Here's how the part is built. I have some questions about the finished solid (model axes, mm). Coordinates: 2 decimals unless noted, no trailing zeros. Order: outer loops, then holes, each group sorted by start corner. A loop starts at its lowest first (then second) coordinate and runs counter-clockwise, first axis right, second up. Notation, with made-up numbers: (16, -29) - (27, -29) arc R32 cw to (27, 0) - close; hole circle Ø11 at (56, 64). An arc over 180 degrees is marked (long way). Answer in a Markdown table with one row per item. Add a question column.
Item 1: I want a section at B-B (x = 0). Please give me the cut outline in (y, z), plus the area to 3 significant figures.
Item 2: I want a section at D-D (y = 1.3). Please give me the cut outline in (x, z).
Item 3: I want a section at A-A (z = 0). Please give me the cut outline in (x, y), plus the area to 3 significant figures.
Item 4: I want a section at C-C (y = 2.6). Please give me the cut outline in (x, z), plus the area to 3 significant figures.
Item 5: If I drill on line 1 along X through (y, z) = (-0.2, 0); line 2 along Z through (x, y) = (0, 1.9), over which ranges is the centre line in solid material (lowest first)? Write a range as from..to.
Item 6: Will this pin go through, and if not, where does the flat tip stop? pin 1 Ø1.5 at (x, y) = (-2.5, 1.5) entering from -Z.
Item 7: Thinking about a two-plate mould opening in X: for faces 1 (the cylindrical face through (-4.88, 3.99, -1.08)), 2 (the flat face through (0, 4, 0)), 3 (the flat face through (-1.2, -0.5, -0.1)), which applies, +X half, -X half, draft (parallel to the pull), parting line (faces both ways), or undercut?
```python
from build123d import *

# Parameters (mm, degrees)
SKETCH1_R            = 5
SKETCH1_R_2          = 1
BOSS_EXTRUDE1_DEPTH  = 4
CUT_SWEEP1_PROFILE_R = 1
SKETCH13_R           = 5
BOSS_EXTRUDE2_DEPTH  = 1
SKETCH14_R           = 5
SKETCH14_R_2         = 1
BOSS_EXTRUDE3_DEPTH  = 0.5


with BuildPart() as part:
    # Sketch1 → Boss-Extrude1 (new body)
    with BuildSketch(Plane(origin=(0, 0, 0), x_dir=(1, 0, 0), z_dir=(0, 1, 0))):
        with Locations(Location((0, 0, 0), (0, 0, 270))):
            Circle(SKETCH1_R)
        with Locations(Location((0, 0, 0), (0, 0, 270))):
            Circle(SKETCH1_R_2, mode=Mode.SUBTRACT)
    extrude(amount=BOSS_EXTRUDE1_DEPTH)

    # Cut-Sweep1: sweep along a path in Sketch2
    with BuildLine(Plane(origin=(0, 2, 0), x_dir=(1, 0, 0), z_dir=(0, 1, 0))) as cut_sweep1_path:
        CenterArc((0, 0), 5, 0, 360)
    # Cut-Sweep1 profile (on start of the path) → Cut-Sweep1 (sweep, cut)
    with BuildSketch(Plane(origin=(5, 2, 0), x_dir=(-1, 0, 0), z_dir=(0, 0, -1))):
        Circle(CUT_SWEEP1_PROFILE_R)
    sweep(path=cut_sweep1_path.line, mode=Mode.SUBTRACT)

    # Sketch13 → Boss-Extrude2 (add)
    with BuildSketch(Plane(origin=(0, 4, 0), x_dir=(1, 0, 0), z_dir=(0, 1, 0))):
        with Locations(Location((0, 0, 0), (0, 0, 270))):
            Circle(SKETCH13_R)
    extrude(amount=BOSS_EXTRUDE2_DEPTH)

    # Sketch14 → Boss-Extrude3 (add)
    with BuildSketch(Plane.XZ):
        with Locations(Location((0, 0, 0), (0, 0, 90))):
            Circle(SKETCH14_R)
        with Locations(Location((0, 0, 0), (0, 0, 270))):
            Circle(SKETCH14_R_2, mode=Mode.SUBTRACT)
    extrude(amount=BOSS_EXTRUDE3_DEPTH)


solid = part.part
```
Values follow:
| question | item | result |
|---|---|---|
| 1 | outline | (-0.5, -5) - (1, -5) arc R1 cw to (3, -5) - (5, -5) - (5, 5) - (3, 5) arc R1 cw to (1, 5) - (-0.5, 5) - (-0.5, 1) - (4, 1) - (4, -1) - (-0.5, -1) - close |
| 1 | area | 42.9 mm^2 |
| 2 | outline | circle Ø8.57 at (0, 0); hole circle Ø2 at (0, 0) |
| 3 | outline | (-5, -0.5) - (-1, -0.5) - (-1, 4) - (1, 4) - (1, -0.5) - (5, -0.5) - (5, 1) arc R1 cw to (5, 3) - (5, 5) - (-5, 5) - (-5, 3) arc R1 cw to (-5, 1) - close |
| 3 | area | 42.9 mm^2 |
| 4 | outline | circle Ø8.4 at (0, 0); hole circle Ø2 at (0, 0) |
| 4 | area | 52.3 mm^2 |
| 5 | line 1 | x = -5..-1, 1..5 |
| 5 | line 2 | z = -4.01..-1, 1..4.01 |
| 6 | pin 1 | stops at z = -4.61 |
| 7 | face 1 | parting line |
| 7 | face 2 | undercut |
| 7 | face 3 | draft |
